Here's how the part is built. I have some questions about the finished solid (model axes, mm). Coordinates: 2 decimals unless noted, no trailing zeros. Loops run counter-clockwise (first coordinate to the right, second up) from the corner with the lowest first, then second, coordinate; pieces in that order, holes last.
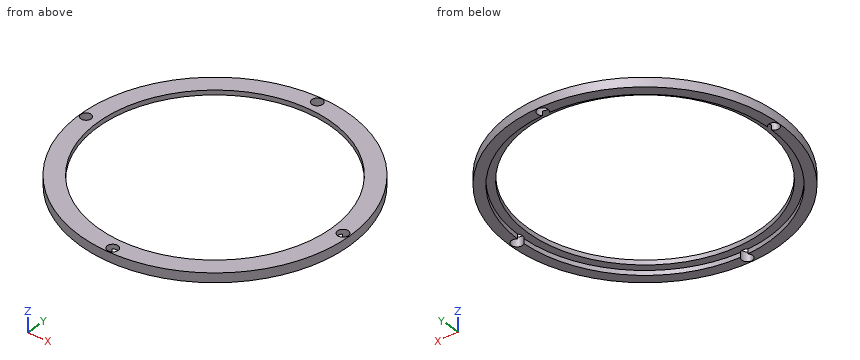
```python
from build123d import *

# Parameters (mm, degrees)
SKETCH016_R     = 58.002282
PAD003_DEPTH    = 4
SKETCH017_R     = 53.661605
POCKET009_DEPTH = 2
SKETCH018_R     = 50.382199
POCKET010_DEPTH = 10
SKETCH019_R     = 2.342621
SKETCH019_R_2   = 2.309522
SKETCH019_R_3   = 2.201756
SKETCH019_R_4   = 2.329825
POCKET011_DEPTH = 5


with BuildPart() as part:
    # Sketch016 → Pad003 (new body)
    with BuildSketch(Plane.XY.offset(100)):
        with Locations((0.009453, 0.01044)):
            Circle(SKETCH016_R)
    extrude(amount=PAD003_DEPTH)

    # Sketch017 → Pocket009 (cut)
    with BuildSketch(Plane(origin=(0, 0, 100), x_dir=(1, 0, 0), z_dir=(0, 0, -1))):
        Circle(SKETCH017_R)
    extrude(amount=-POCKET009_DEPTH, mode=Mode.SUBTRACT)

    # Sketch018 → Pocket010 (cut)
    with BuildSketch(Plane(origin=(0, 0, 102), x_dir=(1, 0, 0), z_dir=(0, 0, -1))):
        Circle(SKETCH018_R)
    extrude(amount=-POCKET010_DEPTH, mode=Mode.SUBTRACT)

    # Sketch019 → Pocket011 (cut)
    with BuildSketch(Plane.XY.offset(104)):
        with Locations((55.227253, -0.025824)):
            Circle(SKETCH019_R)
        with Locations((0.006845, -55.291275)):
            Circle(SKETCH019_R_2)
        with Locations((-55.584568, 0.009231)):
            Circle(SKETCH019_R_3)
        with Locations((-0.004998, 55.371342)):
            Circle(SKETCH019_R_4)
    extrude(amount=-POCKET011_DEPTH, mode=Mode.SUBTRACT)


solid = part.part
```
1. I need wall thicknesses on line 1 along X through (y, z) = (0, 102.6); line 2 along Y through (x, z) = (18, 101.4); line 3 along X through (y, z) = (39.5, 103.7). Which ranges of each line are inside material? Lowest first, please.
2. I want a section at A-A (x = 0). Please give me the cut outline in (y, z), then the cut area to 3 significant figures.
3. For pin 1 (1 mm diameter, centred on y = 27.5, z = 102, fed in from -X); pin 2 (7 mm diameter, centred on x = -55.58, y = 0.01, fed in from -Z); pin 3 (2 mm diameter, centred on x = 31.5, z = 101.5, fed in from +Y), each with a flat end and sliding along its axis, tell me the tip position at first contact or that it passes through.
4. I want a section at B-B (y = 17.5). Please give me the cut outline in (x, z).
5. I want a section at D-D (z = 103). Please give me the cut outline in (x, y) (3 decimals), then the cut area to 3 significant figures.
6. I want a section at C-C (x = -21). Please give me the cut outline in (y, z), then the cut area to 3 significant figures.
Response values:
1. line 1: x = -57.99 to -57.79, -53.38 to -50.38, 50.38 to 52.88, 57.57 to 58.01
1. line 2: y = -55.13 to -50.55, 50.55 to 55.15
1. line 3: x = -42.47 to -31.27, 31.27 to 42.49
2. outline: (-57.99, 100) - (-57.6, 100) - (-57.6, 104) - (-57.99, 104) - close; (-52.98, 102) - (-50.38, 102) - (-50.38, 104) - (-52.98, 104) - close; (50.38, 102) - (53.04, 102) - (53.04, 104) - (50.38, 104) - close; (57.7, 100) - (58.01, 100) - (58.01, 104) - (57.7, 104) - close
2. area: 13.3 mm2
3. pin 1: stops at x = -51.33
3. pin 2: stops at z = 100
3. pin 3: stops at y = 49.35
4. outline: (-55.29, 100) - (-50.73, 100) - (-50.73, 102) - (-47.25, 102) - (-47.25, 104) - (-55.29, 104) - close; (47.25, 102) - (50.73, 102) - (50.73, 100) - (55.31, 100) - (55.31, 104) - (47.25, 104) - close
5. outline: circle Ø116.005 at (0.009, 0.01); hole circle Ø4.404 at (-55.585, 0.009); hole circle Ø100.764 at (0, 0); hole circle Ø4.66 at (-0.005, 55.371); hole circle Ø4.619 at (0.007, -55.291); hole circle Ø4.685 at (55.227, -0.026)
5. area: 2,530 mm2
6. outline: (-54.05, 100) - (-49.38, 100) - (-49.38, 102) - (-45.8, 102) - (-45.8, 104) - (-54.05, 104) - close; (45.8, 102) - (49.38, 102) - (49.38, 100) - (54.07, 100) - (54.07, 104) - (45.8, 104) - close
6. area: 51.8 mm2
